```python
from build123d import *

# Parameters (mm, degrees)
SKETCH_281X300_25_R                    = 2.15
SKETCH_281X300_25_R_2                  = 2.2
SKETCH_281X300_25_R_3                  = 1.6
SKETCH_281X300_25_R_4                  = 1.05
F_4MM_DEPTH                            = 4
FILLET_1_R                             = 8
ELECTRONICS_4X_D3P4_ISO273_OUTLINE_R   = 1.1
ELECTRONICS_4X_D3P4_ISO273_OUTLINE_R_2 = 1.7
ELECTRONICS_4X_D3P4_ISO273_DEPTH       = 4


# Read off the part's stored shape, not the designer's step: Electronics_4x_D3p4_ISO273
with BuildPart() as part:
    # Sketch 281x300__25 → 4mm (new body)
    with BuildSketch(Plane.XY):
        Polygon((-55.5, 150), (-55.5, 99), (-130.5, 99), (-130.5, 57), (-130.5, -57), (-130.5, -99), (-55.5, -99), (-55.5, -150), (57.5, -150), (57.5, -99), (128.5, -99), (128.5, -57), (128.5, 57), (128.5, 99), (57.5, 99), (57.5, 150), align=None)
        with Locations((-44, 140)):
            Circle(SKETCH_281X300_25_R, mode=Mode.SUBTRACT)
        with Locations((26, -140)):
            Circle(SKETCH_281X300_25_R_2, mode=Mode.SUBTRACT)
        with Locations((-24, -140)):
            Circle(SKETCH_281X300_25_R_2, mode=Mode.SUBTRACT)
        with Locations((118.5, 10)):
            Circle(SKETCH_281X300_25_R_3, mode=Mode.SUBTRACT)
        with Locations((118.5, -10)):
            Circle(SKETCH_281X300_25_R_3, mode=Mode.SUBTRACT)
        with Locations((-120.5, 10)):
            Circle(SKETCH_281X300_25_R_3, mode=Mode.SUBTRACT)
        with Locations((-120.5, -10)):
            Circle(SKETCH_281X300_25_R_3, mode=Mode.SUBTRACT)
        with Locations((118.5, 43)):
            Circle(SKETCH_281X300_25_R_3, mode=Mode.SUBTRACT)
        with Locations((118.5, -43)):
            Circle(SKETCH_281X300_25_R_3, mode=Mode.SUBTRACT)
        with Locations((-120.5, 43)):
            Circle(SKETCH_281X300_25_R_3, mode=Mode.SUBTRACT)
        with Locations((-120.5, -43)):
            Circle(SKETCH_281X300_25_R_3, mode=Mode.SUBTRACT)
        with Locations((46, 140)):
            Circle(SKETCH_281X300_25_R, mode=Mode.SUBTRACT)
        with Locations((-44, -140)):
            Circle(SKETCH_281X300_25_R, mode=Mode.SUBTRACT)
        with Locations((46, -140)):
            Circle(SKETCH_281X300_25_R, mode=Mode.SUBTRACT)
        with Locations((-16.5, -45)):
            Circle(SKETCH_281X300_25_R_3, mode=Mode.SUBTRACT)
        with Locations((-106.5, -45)):
            Circle(SKETCH_281X300_25_R_3, mode=Mode.SUBTRACT)
        with Locations((-106.5, 45)):
            Circle(SKETCH_281X300_25_R_3, mode=Mode.SUBTRACT)
        with Locations((-16.5, 45)):
            Circle(SKETCH_281X300_25_R_3, mode=Mode.SUBTRACT)
        with Locations((50.5, -12)):
            Circle(SKETCH_281X300_25_R_3, mode=Mode.SUBTRACT)
        with Locations((95.5, -12)):
            Circle(SKETCH_281X300_25_R_3, mode=Mode.SUBTRACT)
        with Locations((50.5, 47)):
            Circle(SKETCH_281X300_25_R_3, mode=Mode.SUBTRACT)
        with Locations((95.5, 47)):
            Circle(SKETCH_281X300_25_R_3, mode=Mode.SUBTRACT)
        with Locations((3.5, 34.4)):
            Circle(SKETCH_281X300_25_R_4, mode=Mode.SUBTRACT)
        with Locations((28.1, 34.4)):
            Circle(SKETCH_281X300_25_R_4, mode=Mode.SUBTRACT)
        with Locations((3.5, 59.6)):
            Circle(SKETCH_281X300_25_R_4, mode=Mode.SUBTRACT)
        with Locations((28.1, 59.6)):
            Circle(SKETCH_281X300_25_R_4, mode=Mode.SUBTRACT)
    extrude(amount=F_4MM_DEPTH)

    # Fillet 1
    fillet_1_edges = [part.edges().sort_by_distance(p)[0] for p in [
        (-130.5, 99, 2),
        (-55.5, 99, 2),
        (-55.5, 150, 2),
        (57.5, 150, 2),
        (57.5, 99, 2),
        (128.5, 99, 2),
        (128.5, -99, 2),
        (57.5, -99, 2),
        (57.5, -150, 2),
        (-55.5, -150, 2),
        (-55.5, -99, 2),
        (-130.5, -99, 2),
    ]]
    fillet(fillet_1_edges, radius=FILLET_1_R)

    # Electronics_4x_D3p4_ISO273 outline → Electronics_4x_D3p4_ISO273 (cut)
    with BuildSketch(Plane.XY):
        with Locations((-37.3, -78.8)):
            Circle(ELECTRONICS_4X_D3P4_ISO273_OUTLINE_R)
        with Locations((66, -54)):
            Circle(ELECTRONICS_4X_D3P4_ISO273_OUTLINE_R_2)
        with Locations((4, -54)):
            Circle(ELECTRONICS_4X_D3P4_ISO273_OUTLINE_R_2)
        with Locations((-32, -101)):
            Circle(ELECTRONICS_4X_D3P4_ISO273_OUTLINE_R_2)
        with Locations((-12.7, -54.2)):
            Circle(ELECTRONICS_4X_D3P4_ISO273_OUTLINE_R)
        with Locations((-12.7, -78.8)):
            Circle(ELECTRONICS_4X_D3P4_ISO273_OUTLINE_R)
        with Locations((-37.3, -54.2)):
            Circle(ELECTRONICS_4X_D3P4_ISO273_OUTLINE_R)
        with Locations((-32, -126)):
            Circle(ELECTRONICS_4X_D3P4_ISO273_OUTLINE_R_2)
    extrude(amount=ELECTRONICS_4X_D3P4_ISO273_DEPTH, mode=Mode.SUBTRACT)


solid = part.part
```
Work out the finished part from the listing and answer in its coordinate system (mm). Give positions to 0.01 mm unless a question says otherwise; leave off trailing zeros. Loops run counter-clockwise (first coordinate to the right, second up) from the corner with the lowest first, then second, coordinate; pieces in that order, holes last. Notation, with made-up numbers: M 31,43 L 74,43 A18 cw 74,49 Z; hole C -28,64.5 d11. An arc over 180 degrees is marked long. One line per item, written item: value. Start each with the question number.
1. This flat-tipped pin is pushed along its axis until it touches: P1, Ø2, axis at x = 77.5, z = 3, coming from the -Y side. Where does it stop, or does it pass through?
2. Find section B-B (y = 123). Give the vertices of the cut face in (x, z).
3. Find the intervals of material crossed by probe 1 along X at (y, z) = (-78.8, 1.65); probe 2 along Y at (x, z) = (3.5, 1.5); probe 3 along Y at (x, z) = (-12.7, 1.1), in increasing order.
4. Find section A-A (z = 1.7). State how many separate pieces and enclosed holes the cut face has, and give its area (3 significant figures).
Reported:
1. P1: stops at y = -99
2. outline: M -55.5,0 L 57.5,0 L 57.5,4 L -55.5,4 Z
3. probe 1: x = -130.5 to -38.4, -36.2 to -13.8, -11.6 to 128.5
3. probe 2: y = -150 to -55.62, -52.38 to 33.35, 35.45 to 58.55, 60.65 to 150
3. probe 3: y = -150 to -79.9, -77.7 to -55.3, -53.1 to 150
4. separate pieces: 1
4. enclosed holes: 34
4. area: 62,500 mm²
